```python
from build123d import *

# Parameters (mm, degrees)
EXTRUSION1_DEPTH                               = 500
FRAISAGE_POUR_VIS_T_TE_FRAIS_E_M41_D           = 4.5
FRAISAGE_POUR_VIS_T_TE_FRAIS_E_M41_CSINK_D     = 5.5
FRAISAGE_POUR_VIS_T_TE_FRAIS_E_M41_CSINK_ANGLE = 90


with BuildPart() as part:
    # Esquisse1 → Extrusion1 (new body)
    with BuildSketch(Plane.XY):
        with BuildLine():
            Line((-38.885451278, -19.821642953), (-4.885451278, -19.821642953))
            Line((-4.885451278, -19.821642953), (-4.885451278, -15.321642953))
            Line((-4.885451278, -15.321642953), (-14.885451278, -15.321642953))
            Line((-14.885451278, -15.321642953), (-14.885451278, -11.321642953))
            Line((-14.885451278, -11.321642953), (-18.885451278, -4.821642953))
            ThreePointArc((-18.885451278, -4.821642953), (-21.78726352, 6.400322803), (-24.885451278, -4.769021956))
            Line((-24.885451278, -4.769021956), (-28.885451278, -11.321642953))
            Line((-28.885451278, -11.321642953), (-28.885451278, -15.321642953))
            Line((-28.885451278, -15.321642953), (-38.885451278, -15.321642953))
            Line((-38.885451278, -15.321642953), (-38.885451278, -19.821642953))
        make_face()
    extrude(amount=EXTRUSION1_DEPTH)

    # Fraisage pour vis à tête fraisée M41 (through all)
    with Locations(Plane(origin=(-33.885451278, -15.321642953, 50), x_dir=(1, 0, 0), z_dir=(0, 1, 0))):
        with Locations((0, 0), (0, -100), (0, -200), (24, -200), (24, -100), (24, 0), (24, -300), (24, -400), (0, -300), (0, -400)):
            CounterSinkHole(FRAISAGE_POUR_VIS_T_TE_FRAIS_E_M41_D / 2, FRAISAGE_POUR_VIS_T_TE_FRAIS_E_M41_CSINK_D / 2, counter_sink_angle=FRAISAGE_POUR_VIS_T_TE_FRAIS_E_M41_CSINK_ANGLE)


solid = part.part
```
CAD build for the part. Positions are in the model's coordinates, mm. A direction names the side the tool comes from. Coordinates: 2 decimals unless noted, no trailing zeros. Loops run counter-clockwise (first coordinate to the right, second up) from the corner with the lowest first, then second, coordinate; pieces in that order, holes last. Notation, with made-up numbers: (17.5, -34.5) - (46.5, -34.5) arc R29 cw to (46.5, 4.5) - close; hole circle Ø6 at (-2.5, 81.25). An arc over 180 degrees is marked (long way). Use CSV: the item, a comma, the result in double quotes. Start each with the question number.
Q1. Probe probe 1 along X at (y, z) = (-16.95, 350); probe 2 along X at (y, z) = (-15.5, 50.5); probe 3 along Y at (x, z) = (-13.5, 312). List the from-to ranges inside material, lowest first. Write a range as from..to.
Q2. Two-plate mould, pull along Y, no slides. Class faces 1 (the flat face through (-34, -15.322, 246)), 2 (the flat face through (-22, -19.822, 246)), 3 (the flat face through (-22, -9, 500)), 4 (the cylindrical face through (-21.567, 6.394, 246.5)): +Y half, -Y half, draft (parallel to the pull), parting line (faces both ways), or undercut.
Q3. 3-axis set-ups, long thin cutter, end or side, ignore diameter. For faces 5 (the flat face through (-10, -15.322, 246)), 6 (the flat face through (-22, -9, 0)): which of +Z, -Z, +X, -X, +Y, -Y reach the whole face in a straight line?
Q4. Cut at A-A, the plane z = 318. List the corners of the cut face in (x, y), then the cut area to 3 significant figures.
Q5. Drop flat-ended pins along their axis: P1, Ø1, axis at y = 3.5, z = 444.5, coming from the -X side; P2, Ø8, axis at x = -35.5, z = 185.5, coming from the +Y side; P3, Ø5, axis at x = -33.89, z = 150, coming from the +Y side; P4, Ø4, axis at x = -9.89, z = 50, coming from the +Y side. Give the stop position or say it passes through.
Here are the results:
1,probe 1,"-38.89..-36.14, -31.64..-12.14, -7.64..-4.89"
1,probe 2,"-38.89..-36.41, -31.36..-12.41, -7.36..-4.89"
1,probe 3,"-19.82..-15.32"
2,face 1,"+Y half"
2,face 2,"-Y half"
2,face 3,"draft"
2,face 4,"undercut"
3,face 5,"+Z, -Z, +X, +Y"
3,face 6,"-Z, +X, -X, +Y, -Y"
4,outline,"(-38.89, -19.82) - (-4.89, -19.82) - (-4.89, -15.32) - (-14.89, -15.32) - (-14.89, -11.32) - (-18.89, -4.82) arc R6 ccw (long way) to (-24.89, -4.77) - (-28.89, -11.32) - (-28.89, -15.32) - (-38.89, -15.32) - close"
4,area,"384 mm2"
5,P1,"x = -27.25"
5,P2,"y = -15.32"
5,P3,"y = -15.57"
5,P4,"through"
